Verification items for the finished model (mm, model axes). Face numbers are marked on the shaded views. A direction names the side the tool comes from. Coordinates: 2 decimals unless noted, no trailing zeros. Order: outer loops, then holes, each group sorted by start corner. A loop starts at its lowest first (then second) coordinate and runs counter-clockwise, first axis right, second up. Notation, with made-up numbers: M 16.25,23 L 34.25,23 A22 cw 34.25,62 Z; hole C 48,8 d6. An arc over 180 degrees is marked long. Return JSON: item names as keys, results as strings. Group by question number.
1. Section check B-B, the plane z = -1. Record the cut outline in (x, y).
2. Set-up check for the marked faces 1 and 2: record each of +Z, -Z, +X, -X, +Y, -Y from which the full face is reachable in a straight line by a thin tool's end or side.
3. Mould release check, pull along Y, two halves, no side actions. Record for the marked faces 3, 4 and 5: +Y half, -Y half, draft (parallel to the pull), parting line (faces both ways), or undercut.
4. Section check D-D, the plane z = -9.25. Record the cut outline in (x, y), plus the area to 3 significant figures.
5. Gauge pin test, flat ends, axial feed: pin 1 (2.5 mm diameter, centred on x = 1.33, z = 8.4, fed in from +Y); pin 2 (1 mm diameter, centred on x = -3, y = 8.5, fed in from -Z); pin 3 (2 mm diameter, centred on x = 1, y = 3.5, fed in from -Z) (3 decimals). Record the tip position at first contact, or that the pin passes through.
6. Section check C-C, the plane y = 5.5. Record the cut outline in (x, z) (3 decimals), plus the area to 3 significant figures.
7. Section check A-A, the plane x = 0. Record the cut outline in (y, z) (3 decimals).
8. Material ranges on line 1 along Y through (x, z) = (0, -3.5); line 2 along Z through (x, y) = (0, 7.5) (3 decimals); line 3 along X through (y, z) = (1, 0.75), recorded low to high.
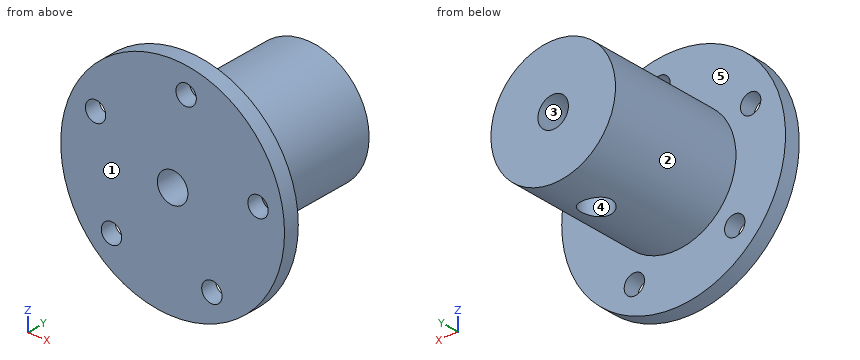
```python
from build123d import *

# Parameters (mm, degrees)
SKIZZE1_R                       = 11
AUFSATZ_LINEAR_AUSTRAGEN1_DEPTH = 1.6
SKIZZE2_R                       = 6.125
AUFSATZ_LINEAR_AUSTRAGEN2_DEPTH = 14
SKIZZE3_R                       = 1.5
SCHNITT_LINEAR_AUSTRAGEN1_DEPTH = 16.6
SKIZZE5_R                       = 0.830846671
SCHNITT_LINEAR_AUSTRAGEN3_DEPTH = 12
SKIZZE8_R                       = 1
SCHNITT_LINEAR_AUSTRAGEN4_DEPTH = 1.6
SKIZZE7_R                       = 1.5
SCHNITT_LINEAR_AUSTRAGEN5_DEPTH = 10


with BuildPart() as part:
    # Skizze1 → Aufsatz-Linear austragen1 (new body)
    with BuildSketch(Plane(origin=(0, 0, 0), x_dir=(1, 0, 0), z_dir=(0, 1, 0))):
        Circle(SKIZZE1_R)
    extrude(amount=AUFSATZ_LINEAR_AUSTRAGEN1_DEPTH)

    # Skizze2 → Aufsatz-Linear austragen2 (add)
    with BuildSketch(Plane(origin=(0, 1.6, 0), x_dir=(1, 0, 0), z_dir=(0, 1, 0))):
        Circle(SKIZZE2_R)
    extrude(amount=AUFSATZ_LINEAR_AUSTRAGEN2_DEPTH)

    # Skizze3 → Schnitt-Linear austragen1 (cut, through all)
    with BuildSketch(Plane(origin=(0, 15.6, 0), x_dir=(1, 0, 0), z_dir=(0, 1, 0))):
        Circle(SKIZZE3_R)
    extrude(amount=-SCHNITT_LINEAR_AUSTRAGEN1_DEPTH, mode=Mode.SUBTRACT)

    # Skizze5 → Schnitt-Linear austragen3 (cut, through all)
    with BuildSketch(Plane.XY):
        with Locations((0, 10.6)):
            Circle(SKIZZE5_R)
    extrude(amount=-SCHNITT_LINEAR_AUSTRAGEN3_DEPTH, mode=Mode.SUBTRACT)

    # Skizze8 → Schnitt-Linear austragen4 (cut)
    with BuildSketch(Plane.XZ):
        with Locations((-6.01040764, -6.01040764)):
            Circle(SKIZZE8_R)
        with Locations((-7.573555456, 3.858919248)):
            Circle(SKIZZE8_R)
        with Locations((1.329692953, 8.395350895)):
            Circle(SKIZZE8_R)
        with Locations((8.395350895, 1.329692953)):
            Circle(SKIZZE8_R)
        with Locations((3.858919248, -7.573555456)):
            Circle(SKIZZE8_R)
    extrude(amount=-SCHNITT_LINEAR_AUSTRAGEN4_DEPTH, mode=Mode.SUBTRACT)

    # Skizze7 → Schnitt-Linear austragen5 (cut)
    with BuildSketch(Plane.XY):
        with Locations((0, 10.6)):
            Circle(SKIZZE7_R)
    extrude(amount=-SCHNITT_LINEAR_AUSTRAGEN5_DEPTH, mode=Mode.SUBTRACT)


solid = part.part
```
Answers follow:
{
 "1": {"outline": "M -10.95,0 L -1.12,0 L -1.12,9.6 A1.5 cw -1.12,11.6 L -1.12,15.6 L -6.04,15.6 L -6.04,1.6 L -10.95,1.6 Z; M 1.12,0 L 10.95,0 L 10.95,1.6 L 6.04,1.6 L 6.04,15.6 L 1.12,15.6 L 1.12,11.6 A1.5 cw 1.12,9.6 Z"},
 "2": {"face 1": "+Z, -Z, +X, -X, -Y", "face 2": "+Y"},
 "3": {"face 3": "draft", "face 4": "undercut", "face 5": "+Y half"},
 "4": {"outline": "M -5.95,0 L 5.95,0 L 5.95,1.6 L -5.95,1.6 Z", "area": "19.0 mm^2"},
 "5": {"pin 1": "y = 1.6", "pin 2": "z = -5.59", "pin 3": "z = -6.125"},
 "6": {"outline": "C 0,0 d12.25; hole C 0,0 d3", "area": "111 mm^2"},
 "7": {"outline": "M 0,-11 L 1.6,-11 L 1.6,-6.125 L 9.1,-6.125 L 9.1,-1.5 L 0,-1.5 Z; M 0,1.5 L 15.6,1.5 L 15.6,6.125 L 1.6,6.125 L 1.6,11 L 0,11 Z; M 12.1,-6.125 L 15.6,-6.125 L 15.6,-1.5 L 12.1,-1.5 Z"},
 "8": {"line 1": "0 to 9.1, 12.1 to 15.6", "line 2": "-6.125 to -1.5, 1.5 to 6.125", "line 3": "-10.97 to -1.3, 1.3 to 7.58, 9.21 to 10.97"}
}
